```python
from build123d import *

# Parameters (mm, degrees)
CROQUIS2_W              = 18
CROQUIS2_H              = 12
CROQUIS2_R              = 1.3
SALIENTE_EXTRUIR1_DEPTH = 6
REDONDEO1_R             = 3


with BuildPart() as part:
    # Croquis2 → Saliente-Extruir1 (new body)
    with BuildSketch(Plane.XY):
        Rectangle(CROQUIS2_W, CROQUIS2_H)
        with Locations((-5.25, 0)):
            Circle(CROQUIS2_R, mode=Mode.SUBTRACT)
        with Locations((5.25, 0)):
            Circle(CROQUIS2_R, mode=Mode.SUBTRACT)
    extrude(amount=SALIENTE_EXTRUIR1_DEPTH)

    # Redondeo1
    redondeo1_edges = [part.edges().sort_by_distance(p)[0] for p in [
        (-9, 6, 3),
        (9, 6, 3),
        (9, -6, 3),
        (-9, -6, 3),
    ]]
    fillet(redondeo1_edges, radius=REDONDEO1_R)


solid = part.part
```
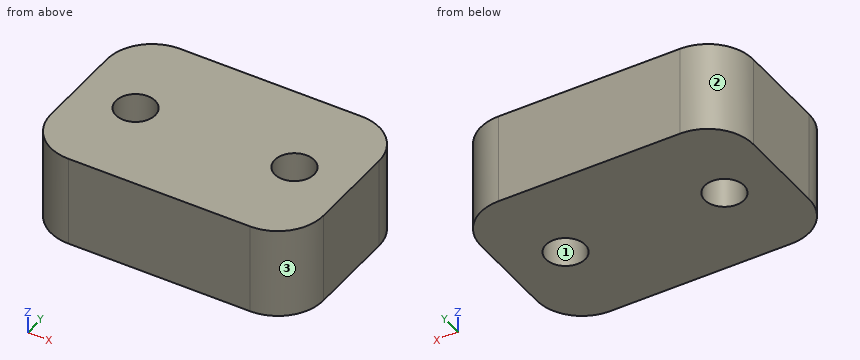
Model file for the job. Use its own axes, mm. Face numbers are marked on the shaded views. Round coordinates to 2 decimals unless told otherwise and drop trailing zeros. Order: outer loops, then holes, each group sorted by start corner. A loop starts at its lowest first (then second) coordinate and runs counter-clockwise, first axis right, second up. Notation, with made-up numbers: M 85.25,39 L 125.25,39 A23 ccw 125.25,54 Z; hole C -12.5,34.5 d6. An arc over 180 degrees is marked long. Use CSV: the item, a comma, the result in double quotes.
Item 1: Pull direction X, two halves, no side cores. Call the marked faces 1, 2 and 3: released by +X, released by -X, zero draft, split by the parting line, or undercut.
Worked answers:
face 1,"undercut"
face 2,"released by -X"
face 3,"released by +X"
Item 2: Saw through at D-D (x = 7.75). List the corners of the cut face in (y, z).
Worked answers:
outline,"M -5.44,0 L 5.44,0 L 5.44,6 L -5.44,6 Z"
Item 3: Saw through at C-C (z = 1.65). List the corners of the cut face in (x, y), plus the area to 3 significant figures.
Worked answers:
outline,"M -9,-3 A3 ccw -6,-6 L 6,-6 A3 ccw 9,-3 L 9,3 A3 ccw 6,6 L -6,6 A3 ccw -9,3 Z; hole C -5.25,0 d2.6; hole C 5.25,0 d2.6"
area,"198 mm²"
Item 4: Pin check, flat tip, straight feed: pin 1 (2 mm diameter, centred on x = -5.25, y = 0, fed in from +Z) (1 decimal). Stop position of the tip, or through.
Worked answers:
pin 1,"through"
Item 5: Probe probe 1 along Y at (x, z) = (5.25, 3); probe 2 along X at (y, z) = (0.25, 4.9); probe 3 along Y at (x, z) = (-6, 5.7). List the from-to ranges inside material, lowest first.
Worked answers:
probe 1,"-6 to -1.3, 1.3 to 6"
probe 2,"-9 to -6.53, -3.97 to 3.97, 6.53 to 9"
probe 3,"-6 to -1.06, 1.06 to 6"
Item 6: Saw through at A-A (x = 5.25). List the corners of the cut face in (y, z).
Worked answers:
outline,"M -6,0 L -1.3,0 L -1.3,6 L -6,6 Z; M 1.3,0 L 6,0 L 6,6 L 1.3,6 Z"
Item 7: Saw through at B-B (y = 0). List the corners of the cut face in (x, z).
Worked answers:
outline,"M -9,0 L -6.55,0 L -6.55,6 L -9,6 Z; M -3.95,0 L 3.95,0 L 3.95,6 L -3.95,6 Z; M 6.55,0 L 9,0 L 9,6 L 6.55,6 Z"
